from build123d import *

# Parameters (mm, degrees)
F0_R     = 11.1125
F0_R_2   = 4.7625
F1_DEPTH = 46.99
F2_W     = 12.7
F2_H     = 3.7792036489
F2_H_2   = 3.4237923279
F3_DEPTH = 3.175
F5_W     = 46.99
F5_H     = 4.4356931467
F6_DEPTH = 25.4
F7_R     = 4.92125
F8_DEPTH = 25.4


# Not quite as in the source:
# - a feature names something its author has since deleted; it is built from what else it names


with BuildPart() as f1:
    # F0 (on Front) → F1 (new body)
    with BuildSketch(Plane.XZ):
        Circle(F0_R)
        Circle(F0_R_2, mode=Mode.SUBTRACT)
    extrude(amount=F1_DEPTH)

    # F2 (on Right) → F3 (join, symmetric)
    with BuildSketch(Plane.YZ):
        with Locations((-40.64, 9.2228981756)):
            Rectangle(F2_W, F2_H)
        with Locations((-6.35, 9.400603836)):
            Rectangle(F2_W, F2_H_2)
    extrude(amount=F3_DEPTH, both=True)

    # F5 (on offset) → F6 (join)
    with BuildSketch(Plane.YZ.offset(9.779)):
        with Locations((-23.495, 0.1773260301)):
            Rectangle(F5_W, F5_H)
    extrude(amount=F6_DEPTH)

    # F7 (on Right) → F8 (cut)
    with BuildSketch(Plane.YZ):
        with Locations((-23.495, 0)):
            Circle(F7_R)
    extrude(amount=-F8_DEPTH, mode=Mode.SUBTRACT)


solid = f1.part
Design review of the part built by this model. Coordinates are the model's own, in mm. A direction names the side the tool comes from. Give positions to 0.01 mm unless a question says otherwise; leave off trailing zeros. Loops run counter-clockwise (first coordinate to the right, second up) from the corner with the lowest first, then second, coordinate; pieces in that order, holes last. Notation, with made-up numbers: (39.5, -18) - (89.5, -18) arc R27 ccw to (89.5, 8) - close; hole circle Ø11 at (31.5, -33.75). An arc over 180 degrees is marked (long way). Write item = value, one per line.
1) Clearance check with flat-ended pins moving along their axes: pin 1 Ø1 at (x, y) = (26.5, -21.5) entering from +Z; pin 2 Ø12 at (x, y) = (28.5, -15.5) entering from -Z; pin 3 Ø5.5 at (x, z) = (0, 0) entering from -Y; pin 4 Ø6 at (y, z) = (-22.5, -6.5) entering from +X. State where each tip first meets the part, or that it passes through.
Result sheet:
pin_1 = 2.4
pin_2 = -2.04
pin_3 = through
pin_4 = 10.55
2) Take a section at B-B on y = -38. State the section outline as (x, z) points (1 decimal), and give its area (3 significant figures).
Result sheet:
outline = (-3.2, 10.6) arc R11.1 ccw (long way) to (10.9, -2) - (35.2, -2) - (35.2, 2.4) - (10.9, 2.4) arc R11.1 ccw to (3.2, 10.6) - (3.2, 11.1) - (-3.2, 11.1) - close; hole circle Ø9.5 at (0, 0)
area = 425 mm2
3) Tool access review of faces 4 (the face through (5, -46.99, 1)), 5 (the face through (-6.71, -28.41, 0.22)), 6 (the face through (35.179, -24, 0)), 7 (the face through (23, -24, -2.041)), 8 (the face through (23, -24, 2.395)): name each direction out of +Z, -Z, +X, -X, +Y, -Y from which nothing blocks a thin tool from reaching the whole face with its end or side.
Result sheet:
face_4 = +Z, -Z, +X, -X, -Y
face_5 = -X
face_6 = +Z, -Z, +X, +Y, -Y
face_7 = -Z, +X, +Y, -Y
face_8 = +Z, +X, +Y, -Y
4) To check wall thickness, follow line 1 (Z direction, x = 0, y = -26); line 2 (X direction, y = -31, z = 0); line 3 (Y direction, x = -5, z = 0). State the ranges of each line that lie inside material, in increasing order.
Result sheet:
line_1 = -11.11 to -4.76, 4.76 to 11.11
line_2 = -11.11 to -4.76, 4.76 to 35.18
line_3 = -46.99 to -28.42, -18.57 to 0
5) Take a section at A-A on z = 0. State the section outline as (x, y) points.
Result sheet:
outline = (-11.11, -46.99) - (-4.76, -46.99) - (-4.76, -28.42) - (-11.11, -28.42) - close; (-11.11, -18.57) - (-4.76, -18.57) - (-4.76, 0) - (-11.11, 0) - close; (4.76, -46.99) - (35.18, -46.99) - (35.18, 0) - (4.76, 0) - close
6) Draft analysis for pull direction Z (two halves, no side actions). For faces 1 (the face through (0, -41, 11.113)), 2 (the face through (4.543, -23.166, 1.431)), 3 (the face through (-3.164, -23.166, -10.653)), state which applies: +Z half, -Z half, draft (parallel to the pull), parting line (faces both ways), or undercut.
Result sheet:
face_1 = +Z half
face_2 = undercut
face_3 = parting line
7) Take a section at D-D on z = -3.5. State the section outline as (x, y) points.
Result sheet:
outline = (-10.55, -46.99) - (-3.23, -46.99) - (-3.23, -26.95) - (-10.55, -26.95) - close; (-10.55, -20.04) - (-3.23, -20.04) - (-3.23, 0) - (-10.55, 0) - close; (3.23, -46.99) - (10.55, -46.99) - (10.55, 0) - (3.23, 0) - close
8) Take a section at C-C on x = -7.5. State the section outline as (y, z) points (1 decimal).
Result sheet:
outline = (-47, -8.2) - (0, -8.2) - (0, 8.2) - (-47, 8.2) - close; hole circle Ø9.8 at (-23.5, 0)
